The figure shows three views and two pictorial views of one solid part (mm, origin at its lowest corner). Answer the questions. Coordinates: 2 decimals unless noted, no trailing zeros. Order: outer loops, then holes, each group sorted by start corner. A loop starts at its lowest first (then second) coordinate and runs counter-clockwise, first axis right, second up. Notation, with made-up numbers: M 37,45.5 L 55,45.5 A23 ccw 55,57.5 Z; hole C -40,33 d6. An arc over 180 degrees is marked long. Use a Markdown table: item, result.
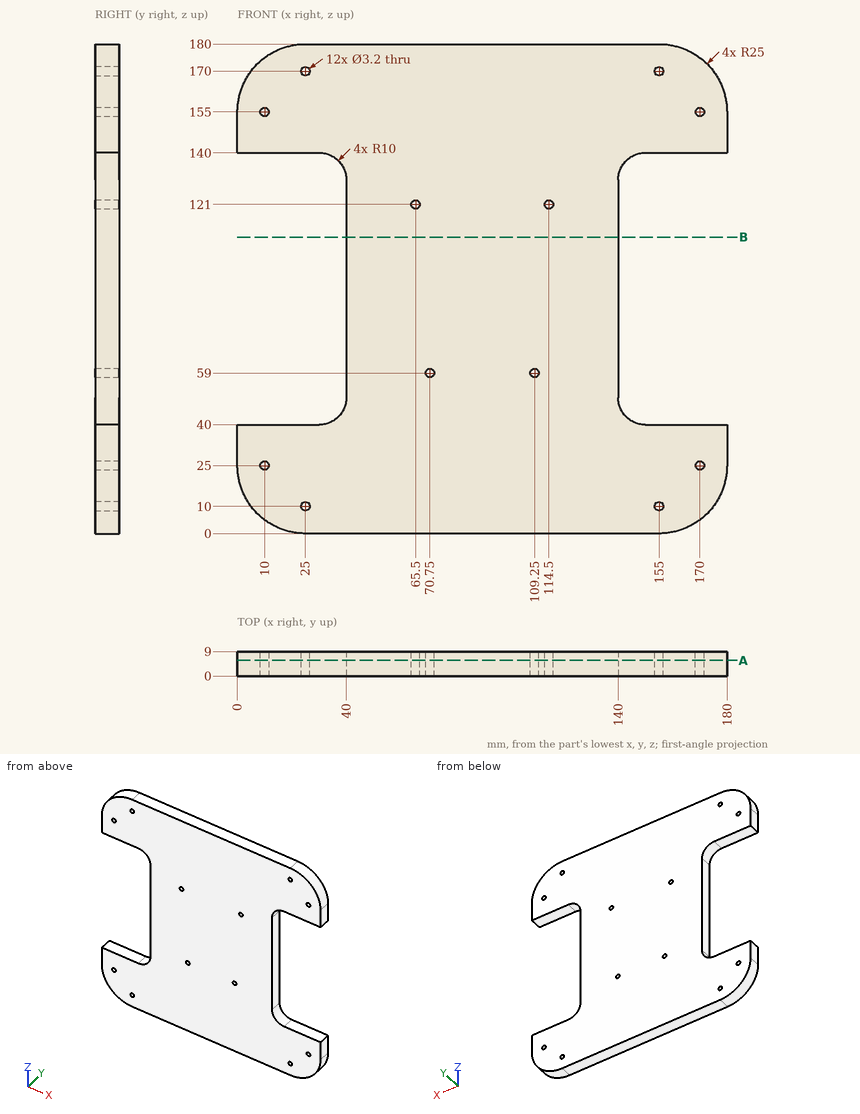
1. Section A-A on y = 5.75 is taken. Give the number of separate pieces and of enclosed holes in the cut face, then the cut area to 3 significant figures.
Answers below:
| item | result |
|---|---|
| separate pieces | 1 |
| enclosed holes | 12 |
| area | 23,900 mm² |
2. Flat-ended cylindrical pins translate along their axes: P1, Ø2.5, axis at x = 159.5, y = 4, coming from the +Z side; P2, Ø4.5, axis at x = 11, y = 2.5, coming from the -Z side; P3, Ø2, axis at y = 7, z = 160, coming from the -X side. Find the tip coordinate at first contact, or state that the pin passes through.
Answers below:
| item | result |
|---|---|
| P1 | z = 179.79 |
| P2 | z = 2.93 |
| P3 | x = 0.32 |
3. Section B-B on z = 109 is taken. Determine the outline of the cut face in (x, y).
Answers below:
| item | result |
|---|---|
| outline | M 40,0 L 140,0 L 140,9 L 40,9 Z |
4. Find the intervals of material crossed by probe 1 along X at (y, z) = (4.5, 59); probe 2 along X at (y, z) = (1.5, 25); probe 3 along Z at (x, y) = (70.75, 7.25), in increasing order.
Answers below:
| item | result |
|---|---|
| probe 1 | 40 to 69.15, 72.35 to 107.65, 110.85 to 140 |
| probe 2 | 0 to 8.4, 11.6 to 168.4, 171.6 to 180 |
| probe 3 | 0 to 57.4, 60.6 to 180 |
